For this review, use the dimensioned drawing (mm, ordinates from the lowest corner) and the shaded views. Give positions to 0.01 mm unless a question says otherwise; leave off trailing zeros. Order: outer loops, then holes, each group sorted by start corner. A loop starts at its lowest first (then second) coordinate and runs counter-clockwise, first axis right, second up. Notation, with made-up numbers: M 66.25,73 L 104.25,73 A10 cw 104.25,91 Z; hole C 85,-6 d6. An arc over 180 degrees is marked long. One line per question, with ' | ' between items. Start each with the question number.
1. The part is to be moulded in two halves that separate along X. For the marked faces 1, 2, 3 and 4, say which applies: +X half, -X half, draft (parallel to the pull), parting line (faces both ways), or undercut.
2. Wall thickness on L1, parallel to Y at x = 55, z = 2.75; L2, parallel to Y at x = 30, z = 2.75: over which ranges is each line inside the solid? List them lowest first.
3. Insertion check: P1, Ø8.5, axis at x = 5, y = 55, coming from the +Z side. The pin has a flat end and moves straight along its axis. Give the tip position at first contact, or say it passes through.
4. We need section B-B on z = 3.5. Write out the cut boundary in (x, y).
5. We need section A-A on y = 5. Write out the cut boundary in (x, z), then the cut area to 3 significant figures.
6. We need section D-D on x = 40. Write out the cut boundary in (y, z).
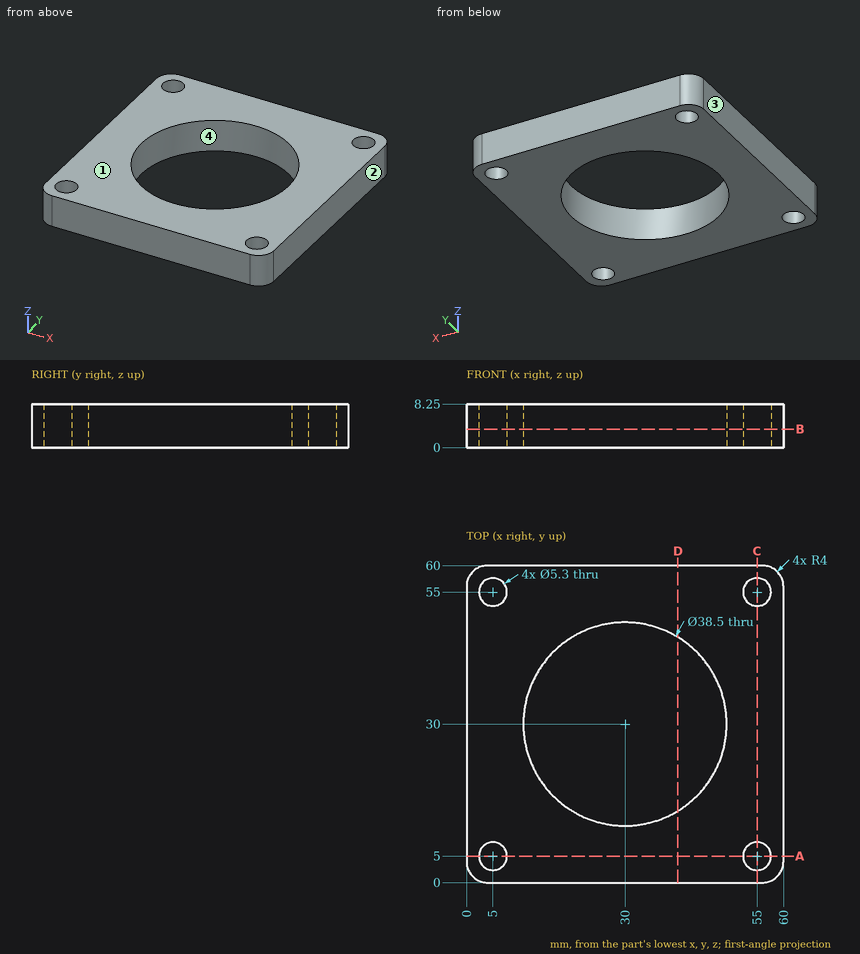
Entries:
1) face 1: draft | face 2: +X half | face 3: -X half | face 4: undercut
2) L1: y = 0 to 2.35, 7.65 to 52.35, 57.65 to 60 | L2: y = 0 to 10.75, 49.25 to 60
3) P1: stops at z = 8.25
4) outline: M 0,4 A4 ccw 4,0 L 56,0 A4 ccw 60,4 L 60,56 A4 ccw 56,60 L 4,60 A4 ccw 0,56 Z; hole C 5,5 d5.3; hole C 5,55 d5.3; hole C 30,30 d38.5; hole C 55,5 d5.3; hole C 55,55 d5.3
5) outline: M 0,0 L 2.35,0 L 2.35,8.25 L 0,8.25 Z; M 7.65,0 L 52.35,0 L 52.35,8.25 L 7.65,8.25 Z; M 57.65,0 L 60,0 L 60,8.25 L 57.65,8.25 Z | area: 408 mm^2
6) outline: M 0,0 L 13.55,0 L 13.55,8.25 L 0,8.25 Z; M 46.45,0 L 60,0 L 60,8.25 L 46.45,8.25 Z
